from build123d import *

# Parameters (mm, degrees)
ESQUISSE1_R             = 10
ESQUISSE1_R_2           = 1.6
BOSS_EXTRU_1_DEPTH      = 2
BOSS_EXTRU_2_DEPTH      = 8
BOSS_EXTRU_2_DEPTH_BACK = 0.0001
ESQUISSE2_R             = 10
ESQUISSE2_R_2           = 1.6
ESQUISSE2_R_3           = 3


with BuildPart() as part:
    # Esquisse1 → Boss.-Extru.1 (new body)
    with BuildSketch(Plane(origin=(0, 0, 0), x_dir=(0, 0, -1), z_dir=(1, 0, 0))):
        Circle(ESQUISSE1_R)
        with Locations((0, 7)):
            Circle(ESQUISSE1_R_2, mode=Mode.SUBTRACT)
        with Locations((7, 0)):
            Circle(ESQUISSE1_R_2, mode=Mode.SUBTRACT)
        with Locations((0, -7)):
            Circle(ESQUISSE1_R_2, mode=Mode.SUBTRACT)
        with Locations((-7, 0)):
            Circle(ESQUISSE1_R_2, mode=Mode.SUBTRACT)
        Circle(ESQUISSE1_R_2, mode=Mode.SUBTRACT)
    extrude(amount=BOSS_EXTRU_1_DEPTH)

    # Esquisse2 → Boss.-Extru.2 (add, two sides: drawn at the far end of the back side and taken through both)
    # profile 1 of 3: a face of its own
    with BuildSketch(Plane(origin=(2, 0, 0), x_dir=(0, 0, -1), z_dir=(1, 0, 0)).offset(-BOSS_EXTRU_2_DEPTH_BACK)):
        Circle(ESQUISSE2_R)
        Circle(ESQUISSE2_R_2, mode=Mode.SUBTRACT)
        with Locations((0, 7)):
            Circle(ESQUISSE2_R_2, mode=Mode.SUBTRACT)
        with Locations((-7, 0)):
            Circle(ESQUISSE2_R_2, mode=Mode.SUBTRACT)
        with Locations((7, 0)):
            Circle(ESQUISSE2_R_2, mode=Mode.SUBTRACT)
        with Locations((0, -7)):
            Circle(ESQUISSE2_R_2, mode=Mode.SUBTRACT)
    # profile 2 of 3: a face of its own
    with BuildSketch(Plane(origin=(2, 0, 0), x_dir=(0, 0, -1), z_dir=(1, 0, 0)).offset(-BOSS_EXTRU_2_DEPTH_BACK)):
        with BuildLine():
            Line((35, 3), (2.017627638, 9.794344221))
            ThreePointArc((2.017627638, 9.794344221), (7.7516539, 6.317583542), (10, 0))
            ThreePointArc((10, 0), (7.7516539, -6.317583542), (2.017627638, -9.794344221))
            Line((2.017627638, -9.794344221), (35, -3))
            ThreePointArc((35, -3), (32, 0), (35, 3))
        make_face()
    # profile 3 of 3: a face of its own
    with BuildSketch(Plane(origin=(2, 0, 0), x_dir=(0, 0, -1), z_dir=(1, 0, 0)).offset(-BOSS_EXTRU_2_DEPTH_BACK)):
        with Locations((35, 0)):
            Circle(ESQUISSE2_R_3)
        with Locations((35, 0)):
            Circle(ESQUISSE2_R_2, mode=Mode.SUBTRACT)
    extrude(amount=BOSS_EXTRU_2_DEPTH + BOSS_EXTRU_2_DEPTH_BACK)


solid = part.part
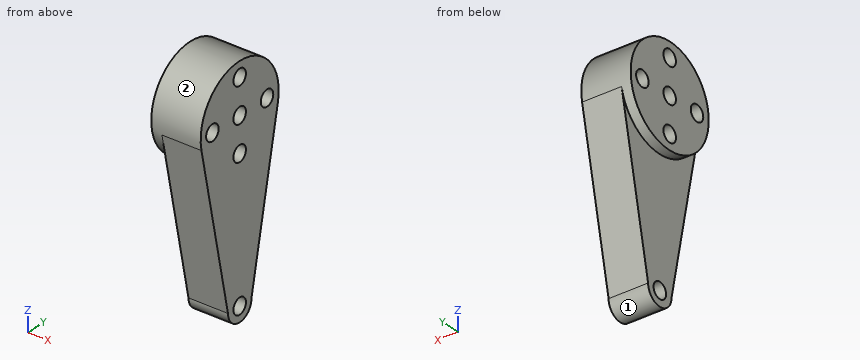
For this review, take the finished solid that the model builds, in its own axes (mm). Face numbers are marked on the shaded views. A direction names the side the tool comes from. Round coordinates to 2 decimals unless told otherwise and drop trailing zeros. Loops run counter-clockwise (first coordinate to the right, second up) from the corner with the lowest first, then second, coordinate; pieces in that order, holes last. Notation, with made-up numbers: (-6.75, -31) - (34.25, -31) arc R16 cw to (34.25, -22) - close; hole circle Ø3 at (66.25, -12). An arc over 180 degrees is marked (long way). Answer as CSV lines item,"result".
(1) Tool access review of the marked faces 1 and 2: name each direction out of +Z, -Z, +X, -X, +Y, -Y from which nothing blocks a thin tool from reaching the whole face with its end or side.
Checked values:
face 1,"-Z, +X, -X"
face 2,"-X"
(2) Consider section D-D on z = -7. Give the boundary of the cut face in (x, y).
Checked values:
outline,"(0, -7.14) - (2, -7.14) - (2, -8.77) - (10, -8.77) - (10, -1.6) - (0, -1.6) - close; (0, 1.6) - (10, 1.6) - (10, 8.77) - (2, 8.77) - (2, 7.14) - (0, 7.14) - close"
(3) Wall thickness on line 1 (Y direction, x = 6, z = 0); line 2 (Z direction, x = 0.5, y = -1); line 3 (Z direction, x = 7, y = -1.25): over which ranges is each line inside the solid? List them lowest first.
Checked values:
line 1,"y = -10 to -8.6, -5.4 to -1.6, 1.6 to 5.4, 8.6 to 10"
line 2,"z = -9.95 to -8.25, -5.75 to -1.25, 1.25 to 5.75, 8.25 to 9.95"
line 3,"z = -37.73 to -36, -34 to -8, -6 to -1, 1 to 6, 8 to 9.92"
(4) Consider section C-C on y = 0. Give the boundary of the cut face in (x, z), then the cut area to 3 significant figures.
Checked values:
outline,"(0, -10) - (2, -10) - (2, -33.4) - (10, -33.4) - (10, -8.6) - (0, -8.6) - close; (0, -5.4) - (10, -5.4) - (10, -1.6) - (0, -1.6) - close; (0, 1.6) - (10, 1.6) - (10, 5.4) - (0, 5.4) - close; (0, 8.6) - (10, 8.6) - (10, 10) - (0, 10) - close; (2, -38) - (10, -38) - (10, -36.6) - (2, -36.6) - close"
area,"302 mm2"
(5) Insertion check: P1, Ø6, axis at y = -1, z = -25, coming from the -X side; P2, Ø1.5, axis at x = 7, y = -1, coming from the +Z side; P3, Ø3, axis at x = 6.5, z = -17.5, coming from the +Y side. Each pin has a flat end and moves straight along its axis. Give the tip position at first contact, or say it passes through.
Checked values:
P1,"stops at x = 2"
P2,"stops at z = 10"
P3,"stops at y = 6.91"
(6) Consider section A-A on z = 0. Give the boundary of the cut face in (x, y).
Checked values:
outline,"(0, -10) - (10, -10) - (10, -8.6) - (0, -8.6) - close; (0, -5.4) - (10, -5.4) - (10, -1.6) - (0, -1.6) - close; (0, 1.6) - (10, 1.6) - (10, 5.4) - (0, 5.4) - close; (0, 8.6) - (10, 8.6) - (10, 10) - (0, 10) - close"
(7) Consider section B-B on x = 7.25. Give the boundary of the cut face in (y, z).
Checked values:
outline,"(-9.79, -2.02) - (-3, -35) arc R3 ccw to (3, -35) - (9.79, -2.02) arc R10 ccw (long way) to start; hole circle Ø3.2 at (-7, 0); hole circle Ø3.2 at (0, -35); hole circle Ø3.2 at (0, -7); hole circle Ø3.2 at (0, 0); hole circle Ø3.2 at (0, 7); hole circle Ø3.2 at (7, 0)"
